Here's how the part is built. I have some questions about the finished solid (model axes, mm). Face numbers are marked on the shaded views. A direction names the side the tool comes from. Give positions to 0.01 mm unless a question says otherwise; leave off trailing zeros. Loops run counter-clockwise (first coordinate to the right, second up) from the corner with the lowest first, then second, coordinate; pieces in that order, holes last. Notation, with made-up numbers: (9.25, 10) - (32.25, 10) arc R19 ccw to (32.25, 47) - close; hole circle Ø2 at (16.5, 14). An arc over 180 degrees is marked (long way). Return JSON: item names as keys, results as strings. Group by question number.
(1) I need wall thicknesses on probe 1 along Y at (x, z) = (10, 0.85) (3 decimals); probe 2 along Z at (x, y) = (1.5, 2). Which ranges of each line are inside material? Lowest first, please. Write a range as [from, to].
(2) On a 3-axis mill with a long thin cutter (end or side, diameter ignored), from which of +Z, -Z, +X, -X, +Y, -Y can I reach the whole of each face in a straight line? I mean the marked faces 1 and 2. Say none if no direction works.
(3) If we section it at B-B (y = -6.75): Please give me the cut outline in (x, z), then the cut area to 3 significant figures.
(4) If we section it at C-C (x = -7.5): Please give me the cut outline in (y, z).
(5) For P1, Ø0.5, axis at x = 11, z = -0.5, coming from the -Y side (3 decimals); P2, Ø5, axis at x = 4.5, y = -8.5, coming from the +Z side; P3, Ø13.5, axis at x = -4.5, y = 4.5, coming from the +Z side; P4, Ø3, axis at x = 10, y = 10, coming from the -Z side, each with a flat end and sliding along its axis, tell me the tip position at first contact or that it passes through.
(6) If we section it at A-A (z = 0.5): Please give me the cut outline in (x, y) (3 decimals), then the cut area to 3 significant figures.
(7) If we section it at D-D (z = 3.35): Please give me the cut outline in (x, y).
```python
from build123d import *

# Parameters (mm, degrees)
F0_W          = 2
F0_H          = 19.25
F1_DEPTH      = 1
F2_R          = 2
F3_D          = 2.25
F4_W          = 8
F4_H          = 5.5
F5_DEPTH      = 3.15
F7_DEPTH      = 2
F7_DEPTH_BACK = 1


with BuildPart() as f1:
    # F0 (on Top) → F1 (new body)
    with BuildSketch(Plane.XY):
        Polygon((13.5, 9.625), (13.5, 13.5), (-13.5, 13.5), (-13.5, 9.625), (-13.5, -9.625), (-13.5, -13.5), (13.5, -13.5), (13.5, -9.625), align=None)
        with Locations((14.5, 0)):
            Rectangle(F0_W, F0_H)
        with Locations((-14.5, 0)):
            Rectangle(F0_W, F0_H)
    extrude(amount=F1_DEPTH)

    # F2
    f2_edges = [f1.edges().sort_by_distance(p)[0] for p in [
        (-13.5, -13.5, 0.5),
        (13.5, -13.5, 0.5),
        (13.5, 13.5, 0.5),
        (-13.5, 13.5, 0.5),
    ]]
    fillet(f2_edges, radius=F2_R)

    # F3 (through all)
    with Locations(Plane(origin=(0, 0, 0), x_dir=(1, 0, 0), z_dir=(0, 0, -1))):
        with Locations((-10, 10), (10, 10), (10, -10), (-10, -10)):
            Hole(F3_D / 2)

    # F4 (on face) → F5 (join)
    with BuildSketch(Plane.XY.offset(1)):
        with Locations((-0.5, -10.75)):
            Rectangle(F4_W, F4_H)
    extrude(amount=F5_DEPTH)

    # F6 (on Top) → F7 (join, two sides)
    with BuildSketch(Plane.XY) as f7_sk:
        with BuildLine():
            Line((-7.875, -13.5), (7.875, -13.5))
            Line((7.875, -13.5), (7.875, -10))
            ThreePointArc((7.875, -10), (8.497398, -8.497398), (10, -7.875))
            Line((10, -7.875), (13.5, -7.875))
            Line((13.5, -7.875), (13.5, 7.875))
            Line((13.5, 7.875), (10, 7.875))
            ThreePointArc((10, 7.875), (8.497398, 8.497398), (7.875, 10))
            Line((7.875, 10), (7.875, 13.5))
            Line((7.875, 13.5), (-7.875, 13.5))
            Line((-7.875, 13.5), (-7.875, 10))
            ThreePointArc((-7.875, 10), (-8.497398, 8.497398), (-10, 7.875))
            Line((-10, 7.875), (-13.5, 7.875))
            Line((-13.5, 7.875), (-13.5, -7.875))
            Line((-13.5, -7.875), (-10, -7.875))
            ThreePointArc((-10, -7.875), (-8.497398, -8.497398), (-7.875, -10))
            Line((-7.875, -10), (-7.875, -13.5))
        make_face()
    extrude(amount=F7_DEPTH)
    extrude(f7_sk.sketch, amount=-F7_DEPTH_BACK)


solid = f1.part
```
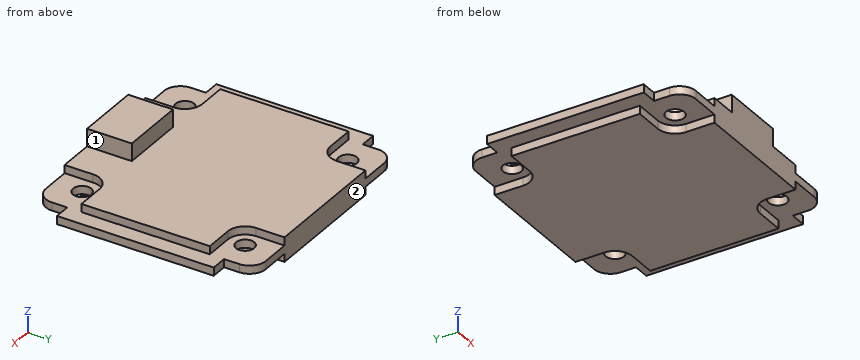
Values:
{
 "1": {"probe 1": "[-13.5, -11.125], [-8.875, 8.875], [11.125, 13.5]", "probe 2": "[-1, 2]"},
 "2": {"face 1": "+Z, +X, +Y, -Y", "face 2": "+Z, -Z, +X, -X, +Y"},
 "3": {"outline": "(-15.5, 0) - (-13.5, 0) - (-13.5, -1) - (13.5, -1) - (13.5, 0) - (15.5, 0) - (15.5, 1) - (13.5, 1) - (13.5, 2) - (-13.5, 2) - (-13.5, 1) - (-15.5, 1) - close", "area": "85.0 mm2"},
 "4": {"outline": "(-13.5, -1) - (13.5, -1) - (13.5, 2) - (-13.5, 2) - close"},
 "5": {"P1": "y = -7.875", "P2": "z = 4.15", "P3": "z = 2", "P4": "z = 0"},
 "6": {"outline": "(-15.5, -9.625) - (-13.5, -9.625) - (-13.5, -11.5) arc R2 ccw to (-11.5, -13.5) - (11.5, -13.5) arc R2 ccw to (13.5, -11.5) - (13.5, -9.625) - (15.5, -9.625) - (15.5, 9.625) - (13.5, 9.625) - (13.5, 11.5) arc R2 ccw to (11.5, 13.5) - (-11.5, 13.5) arc R2 ccw to (-13.5, 11.5) - (-13.5, 9.625) - (-15.5, 9.625) - close; hole circle Ø2.25 at (-10, -10); hole circle Ø2.25 at (-10, 10); hole circle Ø2.25 at (10, -10); hole circle Ø2.25 at (10, 10)", "area": "787 mm2"},
 "7": {"outline": "(-4.5, -13.5) - (3.5, -13.5) - (3.5, -8) - (-4.5, -8) - close"}
}
